CAD build for the part. Positions are in the model's coordinates, mm. A direction names the side the tool comes from. Coordinates: 2 decimals unless noted, no trailing zeros. Order: outer loops, then holes, each group sorted by start corner. A loop starts at its lowest first (then second) coordinate and runs counter-clockwise, first axis right, second up. Notation, with made-up numbers: (40.25, -19) - (92.25, -19) arc R26 cw to (92.25, 17) - close; hole circle Ø11 at (-13, 56). An arc over 180 degrees is marked (long way). Write each question's results on one line, items separated by ' | '. Start each with the question number.
Q1. Band-saw the part on A-A, the plane y = -9. Write the cut outline in (x, z).
Q2. Pin check, flat tips, straight feed: P1, Ø4, axis at x = -2, y = -10.5, coming from the -Z side; P2, Ø2.5, axis at x = 7.5, y = -10.5, coming from the -Z side; P3, Ø4, axis at x = -2.5, y = -13, coming from the +Z side. Stop position of each tip, or through.
Q3. Wall check: probe 1 along Z at (x, y) = (-8, -9); probe 2 along Z at (x, y) = (0, -17.8); probe 3 along Y at (x, z) = (-9.4, -14). Give the ranges that are in metal, low to high.
Q4. Band-saw the part on B-B, the plane z = -14. Write the cut outline in (x, y), then the cut area to 4 significant figures.
Q5. Band-saw the part on D-D, the plane x = -6.5. Write the cut outline in (y, z).
Q6. Pull direction Z, two halves, no side cores. Call faces 4 (the cylindrical face through (-7.46, -17.14, -19.1)), 5 (the flat face through (-2, -17.6, 3)), 6 (the cylindrical face through (-7.54, -17.14, 19.1)): released by +Z, released by -Z, zero draft, split by the parting line, or undercut.
Q7. Which spindle directions (+Z, -Z, +X, -X, +Y, -Y) get a long thin tool onto all of the face, cutting with end or side? Do faces 1 (the cylindrical face through (-5.495, -8.923, 0.235)), 2 (the flat face through (7, -9, -0.5)), 3 (the flat face through (-5, -8.9, -19.4)). Say none if no direction does.
Q8. Band-saw the part on C-C, the plane x = 2. Write the cut outline in (y, z).
```python
from build123d import *
from build123d import SkipClean  # not in build123d's __all__

# Parameters (mm, degrees)
F1_DEPTH       = 18
F2_R           = 5.5
F3_DEPTH       = 18
F5_D           = 5
F5_CSINK_D     = 10
F5_CSINK_ANGLE = 90
F6_W           = 7.3579490118
F6_H           = 1
F7_DEPTH       = 18
F8_R           = 3
F9_R           = 8.5
F9_R_2         = 3
F10_DEPTH      = 0.4


with BuildPart() as f1:
    # F0 (on Front) → F1 (new body)
    with BuildSketch(Plane.XZ):
        with BuildLine():
            ThreePointArc((-5, -6.8738635424), (-8.5, 0), (-5, 6.8738635424))
            Line((-5, 6.8738635424), (-5, 8.5))
            Line((-5, 8.5), (-5, 20))
            Line((-5, 20), (-10, 20))
            Line((-10, 20), (-10, -20))
            Line((-10, -20), (-5, -20))
            Line((-5, -20), (-5, -8.5))
            Line((-5, -8.5), (-5, -6.8738635424))
        make_face()
        with BuildLine():
            ThreePointArc((0, -8.5), (6.0104076401, -6.0104076401), (8.5, 0))
            ThreePointArc((8.5, 0), (6.0104076401, 6.0104076401), (0, 8.5))
            ThreePointArc((0, 8.5), (-2.6288932927, 8.0832493501), (-5, 6.8738635424))
            Line((-5, 6.8738635424), (-5, -6.8738635424))
            ThreePointArc((-5, -6.8738635424), (-2.6288932927, -8.0832493501), (0, -8.5))
        make_face()
        with BuildLine():
            Line((-5, -8.5), (0, -8.5))
            ThreePointArc((0, -8.5), (-2.6288932927, -8.0832493501), (-5, -6.8738635424))
            Line((-5, -6.8738635424), (-5, -8.5))
        make_face()
        with BuildLine():
            Line((-5, -6.8738635424), (-5, 6.8738635424))
            ThreePointArc((-5, 6.8738635424), (-8.5, 0), (-5, -6.8738635424))
        make_face()
        with BuildLine():
            ThreePointArc((-5, 6.8738635424), (-2.6288932927, 8.0832493501), (0, 8.5))
            Line((0, 8.5), (-5, 8.5))
            Line((-5, 8.5), (-5, 6.8738635424))
        make_face()
    extrude(amount=F1_DEPTH)

    # F2 (on face) → F3 (cut, through all)
    with BuildSketch(Plane.XZ.offset(18)):
        Circle(F2_R)
    extrude(amount=-F3_DEPTH, mode=Mode.SUBTRACT)

    # F5 (through all)
    with Locations(Plane.YZ.offset(-5)):
        with Locations((-9, -14), (-9, 14)):
            CounterSinkHole(F5_D / 2, F5_CSINK_D / 2, counter_sink_angle=F5_CSINK_ANGLE)

    # F6 (on Front) → F7 (cut, through all)
    with BuildSketch(Plane.XZ):
        with Locations((7.1057528257, 0)):
            Rectangle(F6_W, F6_H)
    extrude(amount=F7_DEPTH, mode=Mode.SUBTRACT)

    # F8
    f8_edges = [f1.edges().sort_by_distance(p)[0] for p in [
        (-7.5, -18, -20),
        (-7.5, -18, 20),
        (-7.5, 0, 20),
        (-7.5, 0, -20),
    ]]
    fillet(f8_edges, radius=F8_R)

    # F9 (on face) → F10 (join)
    with BuildSketch(Plane.XZ.offset(18)):
        Circle(F9_R)
        Circle(F9_R_2, mode=Mode.SUBTRACT)
    with SkipClean():  # cleaning this boolean's faces spoils the solid; the shape is the same uncleaned
        extrude(amount=-F10_DEPTH)


solid = f1.part
```
Results below:
1) outline: (-10, -20) - (-5, -20) - (-5, -19) - (-7.5, -16.5) - (-10, -16.5) - close; (-10, -11.5) - (-7.5, -11.5) - (-5, -9) - (-5, -8.5) - (0, -8.5) arc R8.5 ccw to (8.49, -0.5) - (5.48, -0.5) arc R5.5 cw (long way) to (5.48, 0.5) - (8.49, 0.5) arc R8.5 ccw to (0, 8.5) - (-5, 8.5) - (-5, 9) - (-7.5, 11.5) - (-10, 11.5) - close; (-10, 16.5) - (-7.5, 16.5) - (-5, 19) - (-5, 20) - (-10, 20) - close
2) P1: stops at z = -8.5 | P2: stops at z = -5.76 | P3: stops at z = 8.5
3) probe 1: z = -20 to -16.5, -11.5 to 11.5, 16.5 to 20 | probe 2: z = -8.5 to -3, 3 to 8.5 | probe 3: y = -18 to -11.5, -6.5 to 0
4) outline: (-10, -18) - (-5, -18) - (-5, -14) - (-7.5, -11.5) - (-10, -11.5) - close; (-10, -6.5) - (-7.5, -6.5) - (-5, -4) - (-5, 0) - (-10, 0) - close | area: 58.75 mm²
5) outline: (-18, -17) arc R3 ccw to (-15, -20) - (-3, -20) arc R3 ccw to (0, -17) - (0, 17) arc R3 ccw to (-3, 20) - (-15, 20) arc R3 ccw to (-18, 17) - close; hole circle Ø7 at (-9, -14); hole circle Ø7 at (-9, 14)
6) face 4: released by -Z | face 5: undercut | face 6: released by +Z
7) face 1: +Y | face 2: +X, +Y | face 3: -Z, +X, +Y, -Y
8) outline: (-18, -8.26) - (0, -8.26) - (0, -5.12) - (-17.6, -5.12) - (-17.6, -2.24) - (-18, -2.24) - close; (-18, 2.24) - (-17.6, 2.24) - (-17.6, 5.12) - (0, 5.12) - (0, 8.26) - (-18, 8.26) - close
